Build history of the part. All positions in model axes, mm. A direction names the side the tool comes from. Give positions to 0.01 mm unless a question says otherwise; leave off trailing zeros. Order: outer loops, then holes, each group sorted by start corner. A loop starts at its lowest first (then second) coordinate and runs counter-clockwise, first axis right, second up. Notation, with made-up numbers: (-34.75, 6.5) -> (9.25, 6.5) arc R25 ccw to (9.25, 30.5) -> close; hole circle Ø11 at (79, -14.5). An arc over 180 degrees is marked (long way). One line per item, written item: value. Start each with the question number.
(1) Saw through at B-B on x = 21.5. Give the cut face in (y, z), plus the area to 3 significant figures.
(2) Two-plate mould, pull along X, no slides. Class faces 1 (the flat face through (16, 2, 0)), 2 (the flat face through (25.4, 2, 125)): +X half, -X half, draft (parallel to the pull), parting line (faces both ways), or undercut.
(3) Probe line 1 (Z direction, x = 8.5, y = 2.45). List the from-to ranges inside material, lowest first.
(4) Which spindle directions (+Z, -Z, +X, -X, +Y, -Y) get a long thin tool onto all of the face, cutting with end or side? Do faces 3 (the flat face through (38.1, 2, 125)), 4 (the flat face through (25, 0, 63)), 5 (the flat face through (6.35, 2, 2)), 6 (the flat face through (48, 2, 3.048)), 7 (the flat face through (29, 2, 127)). Say none if no direction does.
(5) Pin check, flat tips, straight feed: pin 1 (1.5 mm diameter, centred on x = 47, y = 2, fed in from -Z); pin 2 (0.9 mm diameter, centred on y = 1, z = 125, fed in from +X); pin 3 (0.9 mm diameter, centred on x = 8.5, y = 2, fed in from +Z). Stop position of each tip, or through.
```python
from build123d import *

# Parameters (mm, degrees)
BOSS_EXTRUDE1_DEPTH = 3.048


with BuildPart() as part:
    # Sketch1 → Boss-Extrude1 (new body)
    with BuildSketch(Plane(origin=(0, 0, 0), x_dir=(1, 0, 0), z_dir=(0, 1, 0))):
        Polygon((6.35, 0), (0, 0), (0, -63.5), (50.8, -63.5), (50.8, -3.048), (44.45, -3.048), (44.45, 0), (38.1, 0), (38.1, -3.048), (31.75, -3.048), (31.75, 0), (25.4, 0), (25.4, -3.048), (19.05, -3.048), (19.05, 0), (12.7, 0), (12.7, -3.048), (6.35, -3.048), align=None)
        Polygon((50.8, -63.5), (0, -63.5), (0, -127), (6.35, -127), (6.35, -123.952), (12.7, -123.952), (12.7, -127), (19.05, -127), (19.05, -123.952), (25.4, -123.952), (25.4, -127), (31.75, -127), (31.75, -123.952), (38.1, -123.952), (38.1, -127), (44.45, -127), (44.45, -123.952), (50.8, -123.952), align=None)
    extrude(amount=BOSS_EXTRUDE1_DEPTH)


solid = part.part
```
Results below:
1. outline: (0, 3.05) -> (3.05, 3.05) -> (3.05, 123.95) -> (0, 123.95) -> close
1. area: 369 mm²
2. face 1: draft
2. face 2: undercut
3. line 1: z = 3.05 to 123.95
4. face 3: +Z, +Y, -Y
4. face 4: +Z, -Z, +X, -X, -Y
4. face 5: -Z, +Y, -Y
4. face 6: -Z, +X, +Y, -Y
4. face 7: +Z, +X, -X, +Y, -Y
5. pin 1: stops at z = 3.05
5. pin 2: stops at x = 44.45
5. pin 3: stops at z = 123.95
